from build123d import *

# Parameters (mm, degrees)
BOSS_EXTRUDE1_DEPTH = 23
BOSS_EXTRUDE3_DEPTH = 3
BOSS_EXTRUDE4_DEPTH = 9
SKETCH4_R           = 1.7
CUT_EXTRUDE1_DEPTH  = 32.237159536
SKETCH5_W           = 3
SKETCH5_H           = 15
BOSS_EXTRUDE5_DEPTH = 2.85
SKETCH6_R           = 1.6
CUT_EXTRUDE2_DEPTH  = 42.890865789
FILLET1_R           = 2


with BuildPart() as part:
    # Sketch1 → Boss-Extrude1 (new body)
    with BuildSketch(Plane.XY):
        Polygon((0, 0), (-8, 0), (-8, -11), (0, -11), (0, -14), (-11, -14), (-11, 3), (0, 3), align=None)
    extrude(amount=BOSS_EXTRUDE1_DEPTH)

    # Sketch2 → Boss-Extrude3 (add)
    with BuildSketch(Plane.ZY.offset(11)):
        Polygon((23, -14), (0, -14), (-0.138768188, -14.165377487), (15.656319184, -27.419029476), (25.298133329, -15.928362829), align=None)
    extrude(amount=-BOSS_EXTRUDE3_DEPTH)

    # Sketch3 → Boss-Extrude4 (add)
    with BuildSketch(Plane(origin=(-8, 0, 0), x_dir=(0, 0, -1), z_dir=(1, 0, 0))):
        Polygon((-25.298133329, -15.928362829), (-23.383022222, -14.321393805), (-13.741208076, -25.812060452), (-15.656319184, -27.419029476), align=None)
    extrude(amount=BOSS_EXTRUDE4_DEPTH)

    # Sketch4 → Cut-Extrude1 (cut, through all)
    with BuildSketch(Plane(origin=(0, -17.431145721, 20.773630536), x_dir=(-1, 0, 0), z_dir=(0, 0.6427876096865378, -0.7660444431189795))):
        with Locations(Location((3.5, -6.440507181, 0), (0, 0, 90))):
            Circle(SKETCH4_R)
    extrude(amount=-CUT_EXTRUDE1_DEPTH, mode=Mode.SUBTRACT)

    # Sketch5 → Boss-Extrude5 (add)
    with BuildSketch(Plane(origin=(0, -19.038114745, 22.688741644), x_dir=(1, 0, 0), z_dir=(0, -0.6427876096865379, 0.7660444431189792))):
        with Locations((-9.5, -3.440507181)):
            Rectangle(SKETCH5_W, SKETCH5_H)
    extrude(amount=BOSS_EXTRUDE5_DEPTH)

    # Sketch6 → Cut-Extrude2 (cut, through all)
    with BuildSketch(Plane.ZY.offset(11)):
        with Locations((6, -5)):
            Circle(SKETCH6_R)
    extrude(amount=-CUT_EXTRUDE2_DEPTH, mode=Mode.SUBTRACT)

    # Fillet1
    fillet1_edges = [part.edges().sort_by_distance(p)[0] for p in [
        (0, 1.5, 0),
        (0, -12.5, 23),
        (0, 1.5, 23),
        (1, -26.615544964, 14.69876363),
        (1, -15.124878317, 24.340577775),
        (0, -12.5, 0),
    ]]
    fillet(fillet1_edges, radius=FILLET1_R)


solid = part.part
Check sheet for the modelled part. Datum: model origin and axes. Units: mm. A direction names the side the tool comes from. Give positions to 0.01 mm unless a question says otherwise; leave off trailing zeros. Loops run counter-clockwise (first coordinate to the right, second up) from the corner with the lowest first, then second, coordinate; pieces in that order, holes last. Notation, with made-up numbers: M -35,86 L 12,86 A15 cw 12,107 Z; hole C 61,47.5 d7. An arc over 180 degrees is marked long. Answer as a JSON object with one key per item and string values. Group by question number.
Q1. Material ranges on line 1 along Y through (x, z) = (-2.75, 7); line 2 along Y through (x, z) = (-7.5, 18.5); line 3 along X through (y, z) = (-1, 14.25), recorded low to high. Write a range as [from, to].
Q2. Cross-section at C-C on z = 6. Record the cut outline in (x, y).
Q3. Release check for a two-part mould opening along Y. For faces 1 (the cylindrical face through (0.4, -26.19, 15.08)), 2 (the flat face through (-8.4, -5.4, 0)), 3 (the flat face through (-4, 0, 11)) record: released by +Y, released by -Y, zero draft, split by the parting line, or undercut.
Q4. Access from +Z, -Z, +X, -X, +Y, -Y to the whole of each face (thin tool, end or side, straight path). Record for faces 4 (the flat face through (-3.563, -21.754, 20.41)), 5 (the flat face through (-8, -19, 11)), 6 (the cylindrical face through (-0.6, -12.52, 22.43)).
Q5. Go/stop test with flat-tipped pins: P1, Ø6, axis at x = -3, y = -16.5, coming from the -Z side; P2, Ø9.5, axis at y = -17.5, z = 9.5, coming from the +X side; P3, Ø1.9, axis at y = -5, z = 6, coming from the +X side; P4, Ø5.5, axis at y = -7, z = 14.5, coming from the +X side. Record where each tip stops, or that it passes through.
Q6. Cross-section at D-D on x = -4.5. Record the cut outline in (y, z), then the cut area to 3 significant figures.
Q7. Cross-section at B-B on x = -7.5. Record the cut outline in (y, z).
Q8. Cross-section at A-A on y = -5. Record the cut outline in (x, z).
Evaluation:
{
 "1": {"line 1": "y = [-14, -11], [0, 3]", "line 2": "y = [-24.03, -20.14], [-14, -11], [0, 3]", "line 3": "x = [-11, -8]"},
 "2": {"outline": "M -11,-19.32 L -8,-19.32 L -8,-14 L 0,-14 L 0,-11 L -8,-11 L -8,-6.6 L -11,-6.6 Z; M -11,-3.4 L -8,-3.4 L -8,0 L 0,0 L 0,3 L -11,3 Z"},
 "3": {"face 1": "released by -Y", "face 2": "zero draft", "face 3": "undercut"},
 "4": {"face 4": "+Z, +X, -Y", "face 5": "-Z, +X", "face 6": "+Z, +X, +Y"},
 "5": {"P1": "stops at z = 0", "P2": "stops at x = 0", "P3": "passes through", "P4": "stops at x = -8"},
 "6": {"outline": "M -27.42,15.66 L -25.81,13.74 L -23.42,15.75 L -25.02,17.67 Z; M -22.92,19.43 L -21.31,17.52 L -14.32,23.38 L -15.93,25.3 Z; M -14,0 L -11,0 L -11,23 L -14,23 Z; M 0,0 L 3,0 L 3,23 L 0,23 Z", "area": "169 mm2"},
 "7": {"outline": "M -27.42,15.66 L -25.81,13.74 L -14.32,23.38 L -15.93,25.3 Z; M -14,0 L -11,0 L -11,23 L -14,23 Z; M 0,0 L 3,0 L 3,23 L 0,23 Z"},
 "8": {"outline": "M -11,0 L -8,0 L -8,4.4 L -11,4.4 Z; M -11,7.6 L -8,7.6 L -8,23 L -11,23 Z"}
}
